from build123d import *

# Parameters (mm, degrees)
SKETCH1_W           = 311.15
SKETCH1_H           = 79.948192099
BOSS_EXTRUDE1_DEPTH = 1


with BuildPart() as part:
    # Sketch1 → Boss-Extrude1 (new body)
    with BuildSketch(Plane(origin=(0, 0, 0), x_dir=(1, 0, 0), z_dir=(0, 1, 0))):
        with Locations((155.575, 39.97409605)):
            Rectangle(SKETCH1_W, SKETCH1_H)
        with BuildLine():
            Line((16.217864357, 67.248192099), (33.342821045, 67.248192099))
            ThreePointArc((33.342821045, 67.248192099), (34.725807369, 66.44011822), (34.70085023, 64.838552828))
            Line((34.70085023, 64.838552828), (27.77241501, 53.39399889))
            ThreePointArc((27.77241501, 53.39399889), (27.193811945, 52.833151838), (26.414385824, 52.628638162))
            Line((26.414385824, 52.628638162), (23.146299578, 52.628638162))
            ThreePointArc((23.146299578, 52.628638162), (22.366873457, 52.833151838), (21.788270393, 53.39399889))
            Line((21.788270393, 53.39399889), (14.859835172, 64.838552828))
            ThreePointArc((14.859835172, 64.838552828), (14.834878034, 66.44011822), (16.217864357, 67.248192099))
        make_face(mode=Mode.SUBTRACT)
        with BuildLine():
            Line((49.506215761, 67.248192099), (123.456467253, 67.248192099))
            ThreePointArc((123.456467253, 67.248192099), (124.235893374, 67.043678423), (124.814496439, 66.482831371))
            Line((124.814496439, 66.482831371), (139.102316391, 42.881870854))
            ThreePointArc((139.102316391, 42.881870854), (139.273343709, 42.486513094), (139.331787206, 42.059731582))
            Line((139.331787206, 42.059731582), (139.331787206, 37.888460517))
            ThreePointArc((139.331787206, 37.888460517), (139.273343709, 37.461679005), (139.102316391, 37.066321246))
            Line((139.102316391, 37.066321246), (124.814496439, 13.465360728))
            ThreePointArc((124.814496439, 13.465360728), (124.235893374, 12.904513676), (123.456467253, 12.7))
            Line((123.456467253, 12.7), (49.506215761, 12.7))
            ThreePointArc((49.506215761, 12.7), (48.72678964, 12.904513676), (48.148186576, 13.465360728))
            Line((48.148186576, 13.465360728), (33.860366623, 37.066321246))
            ThreePointArc((33.860366623, 37.066321246), (33.689339305, 37.461679005), (33.630895809, 37.888460517))
            Line((33.630895809, 37.888460517), (33.630895809, 42.059731582))
            ThreePointArc((33.630895809, 42.059731582), (33.689339305, 42.486513094), (33.860366623, 42.881870854))
            Line((33.860366623, 42.881870854), (48.148186576, 66.482831371))
            ThreePointArc((48.148186576, 66.482831371), (48.72678964, 67.043678423), (49.506215761, 67.248192099))
        make_face(mode=Mode.SUBTRACT)
        with BuildLine():
            Line((266.056334932, 67.248192099), (283.18129162, 67.248192099))
            ThreePointArc((283.18129162, 67.248192099), (284.564277944, 66.44011822), (284.539320806, 64.838552828))
            Line((284.539320806, 64.838552828), (277.610885585, 53.39399889))
            ThreePointArc((277.610885585, 53.39399889), (277.03228252, 52.833151838), (276.252856399, 52.628638162))
            Line((276.252856399, 52.628638162), (272.984770153, 52.628638162))
            ThreePointArc((272.984770153, 52.628638162), (272.205344032, 52.833151838), (271.626740968, 53.39399889))
            Line((271.626740968, 53.39399889), (264.698305747, 64.838552828))
            ThreePointArc((264.698305747, 64.838552828), (264.673348609, 66.44011822), (266.056334932, 67.248192099))
        make_face(mode=Mode.SUBTRACT)
        with BuildLine():
            Line((16.217864357, 12.7), (33.342821045, 12.7))
            ThreePointArc((33.342821045, 12.7), (34.725807369, 13.508073879), (34.70085023, 15.109639272))
            Line((34.70085023, 15.109639272), (27.77241501, 26.554193209))
            ThreePointArc((27.77241501, 26.554193209), (27.193811945, 27.115040261), (26.414385824, 27.319553938))
            Line((26.414385824, 27.319553938), (23.146299578, 27.319553938))
            ThreePointArc((23.146299578, 27.319553938), (22.366873457, 27.115040261), (21.788270393, 26.554193209))
            Line((21.788270393, 26.554193209), (14.859835172, 15.109639272))
            ThreePointArc((14.859835172, 15.109639272), (14.834878034, 13.508073879), (16.217864357, 12.7))
        make_face(mode=Mode.SUBTRACT)
        with BuildLine():
            Line((139.619861969, 67.248192099), (156.744818657, 67.248192099))
            ThreePointArc((156.744818657, 67.248192099), (158.127804981, 66.44011822), (158.102847842, 64.838552828))
            Line((158.102847842, 64.838552828), (151.174412622, 53.39399889))
            ThreePointArc((151.174412622, 53.39399889), (150.595809557, 52.833151838), (149.816383436, 52.628638162))
            Line((149.816383436, 52.628638162), (146.54829719, 52.628638162))
            ThreePointArc((146.54829719, 52.628638162), (145.768871069, 52.833151838), (145.190268005, 53.39399889))
            Line((145.190268005, 53.39399889), (138.261832784, 64.838552828))
            ThreePointArc((138.261832784, 64.838552828), (138.236875646, 66.44011822), (139.619861969, 67.248192099))
        make_face(mode=Mode.SUBTRACT)
        with BuildLine():
            Line((298.45, 61.560557725), (298.45, 18.387634374))
            ThreePointArc((298.45, 18.387634374), (297.289281512, 16.858577871), (295.504470815, 17.565495103))
            Line((295.504470815, 17.565495103), (283.698837199, 37.066321246))
            ThreePointArc((283.698837199, 37.066321246), (283.52780988, 37.461679005), (283.469366384, 37.888460517))
            Line((283.469366384, 37.888460517), (283.469366384, 42.059731582))
            ThreePointArc((283.469366384, 42.059731582), (283.52780988, 42.486513094), (283.698837199, 42.881870854))
            Line((283.698837199, 42.881870854), (295.504470815, 62.382696997))
            ThreePointArc((295.504470815, 62.382696997), (297.289281512, 63.089614229), (298.45, 61.560557725))
        make_face(mode=Mode.SUBTRACT)
        with BuildLine():
            Line((265.768260169, 37.888460517), (265.768260169, 42.059731582))
            ThreePointArc((265.768260169, 42.059731582), (265.709816672, 42.486513094), (265.538789354, 42.881870854))
            Line((265.538789354, 42.881870854), (251.250969402, 66.482831371))
            ThreePointArc((251.250969402, 66.482831371), (250.672366338, 67.043678423), (249.892940217, 67.248192099))
            Line((249.892940217, 67.248192099), (172.908213373, 67.248192099))
            ThreePointArc((172.908213373, 67.248192099), (172.128787252, 67.043678423), (171.550184188, 66.482831371))
            Line((171.550184188, 66.482831371), (157.262364235, 42.881870854))
            ThreePointArc((157.262364235, 42.881870854), (157.091336917, 42.486513094), (157.032893421, 42.059731582))
            Line((157.032893421, 42.059731582), (157.032893421, 37.888460517))
            ThreePointArc((157.032893421, 37.888460517), (157.091336917, 37.461679005), (157.262364235, 37.066321246))
            Line((157.262364235, 37.066321246), (171.550184188, 13.465360728))
            ThreePointArc((171.550184188, 13.465360728), (172.128787252, 12.904513676), (172.908213373, 12.7))
            Line((172.908213373, 12.7), (249.892940217, 12.7))
            ThreePointArc((249.892940217, 12.7), (250.672366338, 12.904513676), (251.250969402, 13.465360728))
            Line((251.250969402, 13.465360728), (265.538789354, 37.066321246))
            ThreePointArc((265.538789354, 37.066321246), (265.709816672, 37.461679005), (265.768260169, 37.888460517))
        make_face(mode=Mode.SUBTRACT)
        with BuildLine():
            Line((146.54829719, 27.319553938), (149.816383436, 27.319553938))
            ThreePointArc((149.816383436, 27.319553938), (150.595809557, 27.115040261), (151.174412622, 26.554193209))
            Line((151.174412622, 26.554193209), (158.102847842, 15.109639272))
            ThreePointArc((158.102847842, 15.109639272), (158.127804981, 13.508073879), (156.744818657, 12.7))
            Line((156.744818657, 12.7), (139.619861969, 12.7))
            ThreePointArc((139.619861969, 12.7), (138.236875646, 13.508073879), (138.261832784, 15.109639272))
            Line((138.261832784, 15.109639272), (145.190268005, 26.554193209))
            ThreePointArc((145.190268005, 26.554193209), (145.768871069, 27.115040261), (146.54829719, 27.319553938))
        make_face(mode=Mode.SUBTRACT)
        with BuildLine():
            Line((271.626740968, 26.554193209), (264.698305747, 15.109639272))
            ThreePointArc((264.698305747, 15.109639272), (264.673348609, 13.508073879), (266.056334932, 12.7))
            Line((266.056334932, 12.7), (283.18129162, 12.7))
            ThreePointArc((283.18129162, 12.7), (284.564277944, 13.508073879), (284.539320806, 15.109639272))
            Line((284.539320806, 15.109639272), (277.610885585, 26.554193209))
            ThreePointArc((277.610885585, 26.554193209), (277.03228252, 27.115040261), (276.252856399, 27.319553938))
            Line((276.252856399, 27.319553938), (272.984770153, 27.319553938))
            ThreePointArc((272.984770153, 27.319553938), (272.205344032, 27.115040261), (271.626740968, 26.554193209))
        make_face(mode=Mode.SUBTRACT)
    extrude(amount=BOSS_EXTRUDE1_DEPTH)


solid = part.part
Input: part model. Units: mm. Frame: model coordinates. A direction names the side the tool comes from. Give positions to 0.01 mm unless a question says otherwise; leave off trailing zeros. Order: outer loops, then holes, each group sorted by start corner. A loop starts at its lowest first (then second) coordinate and runs counter-clockwise, first axis right, second up.
Q1. Set-up query: faces 4 (the flat face through (153, 0, -41)), 5 (the flat face through (281.124, 0.493, -59.196)). Return all of +Z, -Z, +X, -X, +Y, -Y with unobstructed straight access to the full face (end or side cutting, diameter ignored); none if empty.
Checked values:
face 4: +Z, -Z, +X, -X, -Y
face 5: +Y, -Y
Q2. Draft query along Z for faces 1 (the flat face through (153, 1, -41)), 2 (the flat face through (18.37, 0.49, -20.91)), 3 (the flat face through (31.285, 0.493, -20.752)). Return one class per face: +Z half, -Z half, draft (parallel to the pull), parting line (faces both ways), or undercut.
Checked values:
face 1: draft
face 2: undercut
face 3: undercut
Q3. Section C-C on y = 0.15. State how many separate pieces and enclosed holes the cut face has, and give its area (3 significant figures).
Checked values:
separate pieces: 1
enclosed holes: 9
area: 13,000 mm2
Q4. Section B-B on z = -48.5. Output: boundary loops of the cut face in (x, y), and give its area (3 significant figures).
Checked values:
outline: (0, 0) - (37.26, 0) - (37.26, 1) - (0, 1) - close; (135.7, 0) - (160.66, 0) - (160.66, 1) - (135.7, 1) - close; (262.14, 0) - (287.1, 0) - (287.1, 1) - (262.14, 1) - close; (298.45, 0) - (311.15, 0) - (311.15, 1) - (298.45, 1) - close
area: 99.9 mm2
Q5. Ray query, probe 1 along Z at (x, y) = (276, 0.4); probe 2 along X at (y, z) = (0.65, -40.5); probe 3 along Z at (x, y) = (103.5, 0.4). Return the intervals inside material, ascending.
Checked values:
probe 1: z = -79.95 to -67.25, -52.63 to -27.32, -12.7 to 0
probe 2: x = 0 to 33.63, 139.33 to 157.03, 265.77 to 283.47, 298.45 to 311.15
probe 3: z = -79.95 to -67.25, -12.7 to 0
Q6. Section A-A on x = 106. Output: boundary loops of the cut face in (y, z), and give its area (3 significant figures).
Checked values:
outline: (0, -79.95) - (1, -79.95) - (1, -67.25) - (0, -67.25) - close; (0, -12.7) - (1, -12.7) - (1, 0) - (0, 0) - close
area: 25.4 mm2
